```python
from build123d import *

# Parameters (mm, degrees)
BOSS_EXTRU_1_DEPTH      = 5.5
ENL_V_MAT_EXTRU_1_DEPTH = 0.2


with BuildPart() as part:
    # Esquisse3 → Boss.-Extru.1 (new body)
    with BuildSketch(Plane.XY):
        Polygon((0, 9.6), (9.6, 9.6), (9.6, 0), (2.306440558, 0), (0, 2.306440558), align=None)
    extrude(amount=BOSS_EXTRU_1_DEPTH)

    # Esquisse4 → Enlèv. mat.-Extru.1 (cut)
    with BuildSketch(Plane.XY.offset(5.5)):
        Polygon((4.806969946, 8.146939157), (4.806969946, 9.178990439), (5.12107251, 9.178990439), (5.12107251, 8.146939157), (6.153123792, 8.146939157), (6.153123792, 7.832836593), (5.12107251, 7.832836593), (5.12107251, 6.800785311), (4.806969946, 6.800785311), (4.806969946, 7.832836593), (3.774918664, 7.832836593), (3.774918664, 8.146939157), align=None)
    extrude(amount=-ENL_V_MAT_EXTRU_1_DEPTH, mode=Mode.SUBTRACT)


solid = part.part
```
Can you work these out from the model? Positions are in its coordinate system, mm. Give positions to 0.01 mm unless a question says otherwise; leave off trailing zeros. Order: outer loops, then holes, each group sorted by start corner. A loop starts at its lowest first (then second) coordinate and runs counter-clockwise, first axis right, second up. Notation, with made-up numbers: M -5.5,47.25 L 5.5,47.25 A19 ccw 5.5,84.25 Z; hole C 60,25.25 d1. An arc over 180 degrees is marked long. Write item = value, one per line. Start each with the question number.
Q1. We'd pull the mould along Y, two halves only. Please class faces 1 (the flat face through (5, 9.6, 3)), 2 (the flat face through (5, 8, 5.3)), 3 (the flat face through (0, 6, 3)), 4 (the flat face through (6, 0, 3)): pulls with the +Y half, pulls with the -Y half, needs draft (parallel to the pull), parting line crosses it, or undercut.
Q2. Suppose I cut it at B-B (y = 1). Write out the boundary of the cut face in (x, z), plus the area to 3 significant figures.
Q3. I need wall thicknesses on probe 1 along Y at (x, z) = (2.25, 4.7); probe 2 along X at (y, z) = (0.5, 3.7); probe 3 along Y at (x, z) = (2, 4.85). Which ranges of each line are inside material? Lowest first, please. Write a range as [from, to].
Q4. Suppose I cut it at A-A (z = 2.7). Write out the boundary of the cut face in (x, y), plus the area to 3 significant figures.
Q5. Suppose I cut it at C-C (x = 1.5). Write out the boundary of the cut face in (y, z).
Q6. Will this pin go through, and if not, where does the flat tip stop? pin 1 Ø1 at (x, y) = (4.5, 2.5) entering from -Z.
Check result:
q1.face_1 = pulls with the +Y half
q1.face_2 = undercut
q1.face_3 = needs draft
q1.face_4 = pulls with the -Y half
q2.outline = M 1.31,0 L 9.6,0 L 9.6,5.5 L 1.31,5.5 Z
q2.area = 45.6 mm2
q3.probe_1 = [0.06, 9.6]
q3.probe_2 = [1.81, 9.6]
q3.probe_3 = [0.31, 9.6]
q4.outline = M 0,2.31 L 2.31,0 L 9.6,0 L 9.6,9.6 L 0,9.6 Z
q4.area = 89.5 mm2
q5.outline = M 0.81,0 L 9.6,0 L 9.6,5.5 L 0.81,5.5 Z
q6.pin_1 = 0
